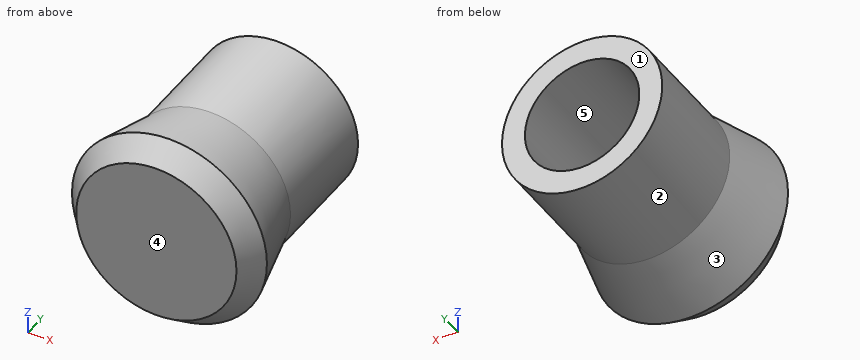
from build123d import *

# Parameters (mm, degrees)
SKETCH001_R  = 7
SKETCH_R     = 9
PAD_DEPTH    = 10
SKETCH002_R  = 5
POCKET_DEPTH = 17
CHAMFER_SIZE = 2


with BuildPart() as part:
    # Sketch001 → AdditiveLoft section 0
    with BuildSketch(Plane.XZ.offset(-8)):
        Circle(SKETCH001_R)
    # Sketch → AdditiveLoft section 1
    with BuildSketch(Plane.XZ):
        Circle(SKETCH_R)
    loft()

    # Sketch001 → Pad (new body)
    with BuildSketch(Plane.XZ.offset(-8)):
        Circle(SKETCH001_R)
    extrude(amount=-PAD_DEPTH)

    # Sketch002 (on Face4 of Pad) → Pocket (cut)
    with BuildSketch(Plane(origin=(0, 18, 0), x_dir=(1, 0, 0), z_dir=(0, 1, 0))):
        Circle(SKETCH002_R)
    extrude(amount=-POCKET_DEPTH, mode=Mode.SUBTRACT)

    # Chamfer
    chamfer_edges = [part.edges().sort_by_distance(p)[0] for p in [
        (-9, 0, 0),
    ]]
    chamfer(chamfer_edges, length=CHAMFER_SIZE)


solid = part.part
The model under review builds one solid part; all positions refer to its coordinate system, in mm. Face numbers are marked on the shaded views. A direction names the side the tool comes from. Coordinates: 2 decimals unless noted, no trailing zeros. Loops run counter-clockwise (first coordinate to the right, second up) from the corner with the lowest first, then second, coordinate; pieces in that order, holes last. Notation, with made-up numbers: (7.25, 88.25) -> (55.25, 88.25) arc R8 ccw to (55.25, 100.25) -> close; hole circle Ø8 at (84, -34.75). An arc over 180 degrees is marked (long way). Use a Markdown table: item, result. Add a question column.
1. To check wall thickness, follow line 1 (Z direction, x = 0, y = 14.25); line 2 (Y direction, x = 1.75, z = -2); line 3 (Z direction, x = 2.75, y = 1.25). State the ranges of each line that lie inside material, in increasing order.
2. Draft analysis for pull direction X (two halves, no side actions). For the marked faces 3, 4 and 5, state which applies: pulls with the +X half, pulls with the -X half, needs draft (parallel to the pull), parting line crosses it, or undercut.
3. Add section A-A on x = 0. Write out the cut boundary in (y, z).
4. Add section B-B on y = 9.5. Write out the cut boundary in (x, z), plus the area to 3 significant figures.
5. Clearance check with flat-ended pins moving along their axes: pin 1 Ø6 at (x, y) = (-2, 13.5) entering from +Z; pin 2 Ø5 at (x, y) = (-6.5, 9.5) entering from +Z; pin 3 Ø2 at (y, z) = (4.5, -1.5) entering from -X. State where each tip first meets the part, or that it passes through.
6. Machinability: for the marked faces 1 and 2, which of the approach directions +Z, -Z, +X, -X, +Y, -Y give a long, thin tool a straight path to every point of the face, cutting with its end or side? Answer none if there is none.
Returned:
| question | item | result |
|---|---|---|
| 1 | line 1 | z = -7 to -5, 5 to 7 |
| 1 | line 2 | y = 0 to 1 |
| 1 | line 3 | z = -7.49 to -4.18, 4.18 to 7.49 |
| 2 | face 3 | parting line crosses it |
| 2 | face 4 | needs draft |
| 2 | face 5 | undercut |
| 3 | outline | (0, -7) -> (1.94, -8.51) -> (8, -7) -> (18, -7) -> (18, -5) -> (1, -5) -> (1, 5) -> (18, 5) -> (18, 7) -> (8, 7) -> (1.94, 8.51) -> (0, 7) -> close |
| 4 | outline | circle Ø14 at (0, 0); hole circle Ø10 at (0, 0) |
| 4 | area | 75.4 mm² |
| 5 | pin 1 | stops at z = 7 |
| 5 | pin 2 | stops at z = 5.74 |
| 5 | pin 3 | stops at x = -8.03 |
| 6 | face 1 | +Z, -Z, +X, -X, +Y |
| 6 | face 2 | +Y |
